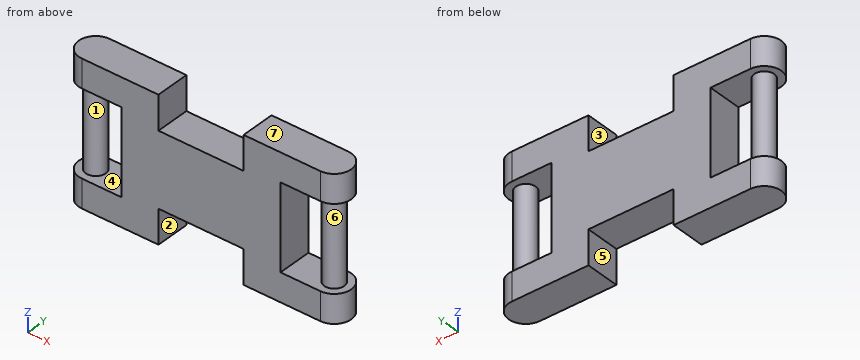
from build123d import *

# Parameters (mm, degrees)
BOSS_EXTRUDE1_DEPTH = 125
SKETCH2_W           = 35
SKETCH2_H           = 75
SKETCH2_W_2         = 15
CUT_EXTRUDE1_DEPTH  = 100
SKETCH3_R           = 8.75
BOSS_EXTRUDE2_DEPTH = 75
SKETCH4_W           = 75
SKETCH4_H           = 30
CUT_EXTRUDE2_DEPTH  = 176.855053951


with BuildPart() as part:
    # Sketch1 → Boss-Extrude1 (new body)
    with BuildSketch(Plane.XY):
        with BuildLine():
            Line((-105, 15), (105, 15))
            ThreePointArc((105, 15), (120, 0), (105, -15))
            Line((105, -15), (-105, -15))
            ThreePointArc((-105, -15), (-120, 0), (-105, 15))
        make_face()
    extrude(amount=BOSS_EXTRUDE1_DEPTH)

    # Sketch2 → Cut-Extrude1 (cut)
    with BuildSketch(Plane(origin=(0, 15, 0), x_dir=(1, 0, 0), z_dir=(0, 1, 0))):
        with Locations((-87.5, -62.5)):
            Rectangle(SKETCH2_W, SKETCH2_H)
        with Locations((-112.5, -62.5)):
            Rectangle(SKETCH2_W_2, SKETCH2_H)
        with Locations((112.5, -62.5)):
            Rectangle(SKETCH2_W_2, SKETCH2_H)
        with Locations((87.5, -62.5)):
            Rectangle(SKETCH2_W, SKETCH2_H)
    extrude(amount=-CUT_EXTRUDE1_DEPTH, mode=Mode.SUBTRACT)

    # Sketch3 → Boss-Extrude2 (add)
    with BuildSketch(Plane.XY.offset(25)):
        with Locations(Location((-105, 0, 0), (0, 0, 180))):
            Circle(SKETCH3_R)
        with Locations(Location((105, 0, 0), (0, 0, 180))):
            Circle(SKETCH3_R)
    extrude(amount=BOSS_EXTRUDE2_DEPTH)

    # Sketch4 → Cut-Extrude2 (cut, through all)
    with BuildSketch(Plane(origin=(0, 15, 0), x_dir=(1, 0, 0), z_dir=(0, 1, 0))):
        with Locations((0, -15)):
            Rectangle(SKETCH4_W, SKETCH4_H)
        with Locations((0, -110)):
            Rectangle(SKETCH4_W, SKETCH4_H)
    extrude(amount=-CUT_EXTRUDE2_DEPTH, mode=Mode.SUBTRACT)


solid = part.part
Geometry: final body of the model. Coordinates: model frame, mm. Face numbers are marked on the shaded views. A direction names the side the tool comes from. Round coordinates to 2 decimals unless told otherwise and drop trailing zeros. Loops run counter-clockwise (first coordinate to the right, second up) from the corner with the lowest first, then second, coordinate; pieces in that order, holes last. Notation, with made-up numbers: (86.25, -17.75) - (127.25, -17.75) arc R25 cw to (127.25, 9.25) - close; hole circle Ø3 at (33, 59.25). An arc over 180 degrees is marked (long way). Write each question's results on one line, items separated by ' | '. Start each with the question number.
1) Mould query, pull axis Z, two halves, no side actions, for the marked faces 4, 5, 6 and 7. Classes: released by +Z, released by -Z, zero draft, split by the parting line, or undercut.
2) Cut plane B-B on z = 110.5. Return loops of the section in (x, y).
3) Line query: probe 1 along Z at (x, y) = (-83, 11); probe 2 along X at (y, z) = (8, 66); probe 3 along Z at (x, y) = (23.5, -9.5). Output: solid intervals per line, ascending. Write a range as [from, to].
4) First-contact query: P1, Ø9, axis at x = 4, y = 5.5, coming from the +Z side; P2, Ø15, axis at x = 86, y = -0.5, coming from the -Z side; P3, Ø4, axis at y = -6, z = 92.5, coming from the -X side; P4, Ø12, axis at y = 6.5, z = 40.5, coming from the -X side. Flat tips, straight axial feed; report the tip coordinate or a pass-through.
5) Access query for the marked faces 1, 2 and 3. Directions: +Z, -Z, +X, -X, +Y, -Y. A direction counts if a zero-diameter tool reaches every point of the face in a straight line with its end or side. Return the directions, or none.
6) Cut plane C-C on z = 47. Return loops of the section in (x, y).
7) Cut plane D-D on y = 0. Return loops of the section in (x, z), then the cut area to 3 significant figures.
8) Cut plane A-A on x = -79.5. Return loops of the section in (y, z), then the cut area to 3 significant figures.
Verdict:
1) face 4: undercut | face 5: zero draft | face 6: undercut | face 7: released by +Z
2) outline: (-105, -15) - (-37.5, -15) - (-37.5, 15) - (-105, 15) arc R15 ccw to start; (37.5, -15) - (105, -15) arc R15 ccw to (105, 15) - (37.5, 15) - close
3) probe 1: z = [0, 25], [100, 125] | probe 2: x = [-108.54, -101.46], [-70, 70], [101.46, 108.54] | probe 3: z = [30, 95]
4) P1: stops at z = 95 | P2: stops at z = 0 | P3: stops at x = -112.78 | P4: stops at x = -113.74
5) face 1: none | face 2: -Z, +Y, -Y | face 3: +Z, +Y, -Y
6) outline: circle Ø17.5 at (-105, 0); (-70, -15) - (70, -15) - (70, 15) - (-70, 15) - close; circle Ø17.5 at (105, 0)
7) outline: (-120, 0) - (-37.5, 0) - (-37.5, 30) - (37.5, 30) - (37.5, 0) - (120, 0) - (120, 25) - (113.75, 25) - (113.75, 100) - (120, 100) - (120, 125) - (37.5, 125) - (37.5, 95) - (-37.5, 95) - (-37.5, 125) - (-120, 125) - (-120, 100) - (-113.75, 100) - (-113.75, 25) - (-120, 25) - close; hole (-96.25, 25) - (-70, 25) - (-70, 100) - (-96.25, 100) - close; hole (70, 25) - (96.25, 25) - (96.25, 100) - (70, 100) - close | area: 20,600 mm2
8) outline: (-15, 0) - (15, 0) - (15, 25) - (-15, 25) - close; (-15, 100) - (15, 100) - (15, 125) - (-15, 125) - close | area: 1,500 mm2
